from build123d import *

# Parameters (mm, degrees)
SALIENTE_EXTRUIR1_DEPTH = 20
CROQUIS2_R              = 30
CORTAR_EXTRUIR1_DEPTH   = 21
CROQUIS3_R              = 10
CORTAR_EXTRUIR2_DEPTH   = 21
CROQUIS4_R              = 10
SALIENTE_EXTRUIR2_DEPTH = 20


with BuildPart() as part:
    # Croquis1 → Saliente-Extruir1 (new body)
    with BuildSketch(Plane(origin=(0, 0, 0), x_dir=(1, 0, 0), z_dir=(0, 1, 0))):
        with BuildLine():
            ThreePointArc((70, -17.320508076), (100, 0), (70, 17.320508076))
            ThreePointArc((70, 17.320508076), (49.330532905, 13.841855007), (31.428571429, 24.743582965))
            ThreePointArc((31.428571429, 24.743582965), (0, 40), (-31.428571429, 24.743582965))
            ThreePointArc((-31.428571429, 24.743582965), (-49.330532905, 13.841855007), (-70, 17.320508076))
            ThreePointArc((-70, 17.320508076), (-100, 0), (-70, -17.320508076))
            ThreePointArc((-70, -17.320508076), (-49.330532905, -13.841855007), (-31.428571429, -24.743582965))
            ThreePointArc((-31.428571429, -24.743582965), (0, -40), (31.428571429, -24.743582965))
            ThreePointArc((31.428571429, -24.743582965), (49.330532905, -13.841855007), (70, -17.320508076))
        make_face()
    extrude(amount=SALIENTE_EXTRUIR1_DEPTH)

    # Croquis2 → Cortar-Extruir1 (cut, through all)
    with BuildSketch(Plane(origin=(0, 20, 0), x_dir=(1, 0, 0), z_dir=(0, 1, 0))):
        Circle(CROQUIS2_R)
    extrude(amount=-CORTAR_EXTRUIR1_DEPTH, mode=Mode.SUBTRACT)

    # Croquis3 → Cortar-Extruir2 (cut, through all)
    with BuildSketch(Plane(origin=(0, 20, 0), x_dir=(1, 0, 0), z_dir=(0, 1, 0))):
        with Locations((-80, 0)):
            Circle(CROQUIS3_R)
    extrude(amount=-CORTAR_EXTRUIR2_DEPTH, mode=Mode.SUBTRACT)

    # Croquis4 → Saliente-Extruir2 (add)
    with BuildSketch(Plane(origin=(0, 20, 0), x_dir=(1, 0, 0), z_dir=(0, 1, 0))):
        with Locations((80, 0)):
            Circle(CROQUIS4_R)
    extrude(amount=SALIENTE_EXTRUIR2_DEPTH)


solid = part.part
Build history of the part. All positions in model axes, mm. A direction names the side the tool comes from. Give positions to 0.01 mm unless a question says otherwise; leave off trailing zeros. Order: outer loops, then holes, each group sorted by start corner. A loop starts at its lowest first (then second) coordinate and runs counter-clockwise, first axis right, second up. Notation, with made-up numbers: M -12.5,82.5 L 11.5,82.5 A22 cw 11.5,115.5 Z; hole C 68.5,27 d2. An arc over 180 degrees is marked long. Put each result on its own line as item: value.
Item 1: Two-plate mould, pull along X, no slides. Class faces 1 (the cylindrical face through (99.99, 9.86, 0.59)), 2 (the flat face through (29, 0, -9)), 3 (the cylindrical face through (-0.506, 9.86, 39.997)): +X half, -X half, draft (parallel to the pull), parting line (faces both ways), or undercut.
From the geometry:
face 1: undercut
face 2: draft
face 3: parting line
Item 2: Slice it at A-A, the plane z = 0. Write the cut outline in (x, y), plus the area to 3 significant figures.
From the geometry:
outline: M -100,0 L -90,0 L -90,20 L -100,20 Z; M -70,0 L -30,0 L -30,20 L -70,20 Z; M 30,0 L 100,0 L 100,20 L 90,20 L 90,40 L 70,40 L 70,20 L 30,20 Z
area: 2,800 mm2
Item 3: Slice it at B-B, the plane x = -80. Write the cut outline in (y, z).
From the geometry:
outline: M 0,-20 L 20,-20 L 20,-10 L 0,-10 Z; M 0,10 L 20,10 L 20,20 L 0,20 Z
Item 4: 3-axis set-ups, long thin cutter, end or side, ignore diameter. For faces 4 (the cylindrical face through (70, 30, 0)), 5 (the flat face through (80, 40, 0)): which of +Z, -Z, +X, -X, +Y, -Y reach the whole face in a straight line?
From the geometry:
face 4: +Y
face 5: +Z, -Z, +X, -X, +Y
Item 5: Slice it at D-D, the plane y = 10. Write the cut outline in (x, z).
From the geometry:
outline: M -70,-17.32 A30 cw -31.43,-24.74 A40 ccw 31.43,-24.74 A30 cw 70,-17.32 A20 ccw long 70,17.32 A30 cw 31.43,24.74 A40 ccw -31.43,24.74 A30 cw -70,17.32 A20 ccw long Z; hole C -80,0 d20; hole C 0,0 d60
Item 6: Probe line 1 (X direction, y = 7.5, z = -8.5); line 2 (Z direction, x = -80, y = 13); line 3 (Z direction, x = 0, y = 11.75). List the from-to ranges inside material, lowest first. Write a range as [from, to].
From the geometry:
line 1: x = [-98.1, -85.27], [-74.73, -28.77], [28.77, 98.1]
line 2: z = [-20, -10], [10, 20]
line 3: z = [-40, -30], [30, 40]
Item 7: Slice it at C-C, the plane x = 80. Write the cut outline in (y, z).
From the geometry:
outline: M 0,-20 L 20,-20 L 20,-10 L 40,-10 L 40,10 L 20,10 L 20,20 L 0,20 Z
Item 8: Flat gauge pins, fed straight in: pin 1 Ø1.5 at (y, z) = (29, 5.5) entering from +X; pin 2 Ø24 at (x, z) = (-27.5, 18) entering from +Y; pin 3 Ø5 at (y, z) = (21, 29.5) entering from +X. Where does each tip first touch, or does it go through?
From the geometry:
pin 1: stops at x = 88.8
pin 2: stops at y = 20
pin 3: stops at x = 29.32
